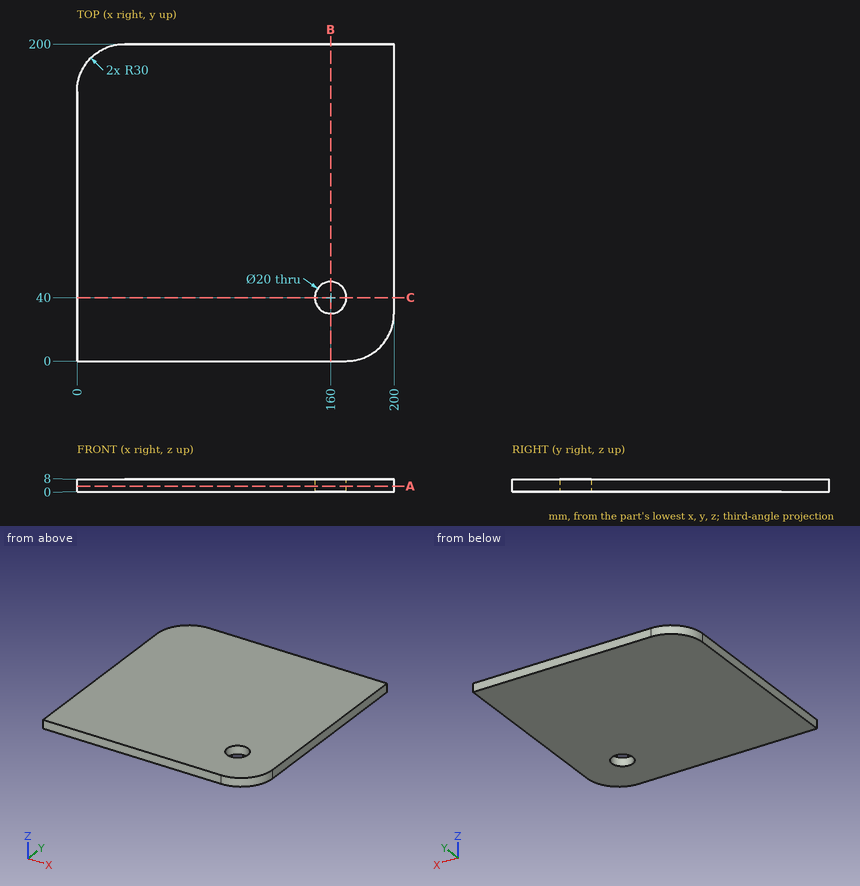
Geometry: see drawing. Coordinates: mm, zero at the bounding-box minimum. Round coordinates to 2 decimals unless told otherwise and drop trailing zeros. Write each loop counter-clockwise with the first axis right and the second up, starting at its lowest first coordinate (ties: lowest second). Pieces come first, ordered by that corner, then holes.
Item 1: Section query C-C (y = 40). Return loops of the section in (x, z), plus the area to 3 significant figures.
Item 2: Section query B-B (x = 160). Return loops of the section in (y, z), plus the area to 3 significant figures.
Item 3: Section query A-A (z = 3.5). Return loops of the section in (x, y).
Item 4: Material intervals for L1, parallel to Y at x = 160, z = 4.5; L2, parallel to X at y = 39.5, z = 1; L3, parallel to X at y = 39, z = 6.5, sorted ascending.
Item 5: Pin query (flat end, axial travel): P1, Ø16, axis at x = 160, y = 40, coming from the +Z side. Return the tip coordinate at first contact, or that it passes through.
Completed:
1. outline: (0, 0) - (150, 0) - (150, 8) - (0, 8) - close; (170, 0) - (200, 0) - (200, 8) - (170, 8) - close
1. area: 1,440 mm2
2. outline: (0, 0) - (30, 0) - (30, 8) - (0, 8) - close; (50, 0) - (200, 0) - (200, 8) - (50, 8) - close
2. area: 1,440 mm2
3. outline: (0, 0) - (170, 0) arc R30 ccw to (200, 30) - (200, 200) - (30, 200) arc R30 ccw to (0, 170) - close; hole circle Ø20 at (160, 40)
4. L1: y = 0 to 30, 50 to 200
4. L2: x = 0 to 150.01, 169.99 to 200
4. L3: x = 0 to 150.05, 169.95 to 200
5. P1: passes through
